Verification items for the finished model (mm, model axes). Face numbers are marked on the shaded views. A direction names the side the tool comes from. Coordinates: 2 decimals unless noted, no trailing zeros. Write each loop counter-clockwise with the first axis right and the second up, starting at its lowest first coordinate (ties: lowest second). Pieces come first, ordered by that corner, then holes. Notation, with made-up numbers: (85, 82.5) -> (126, 82.5) arc R21 cw to (126, 121.5) -> close; hole circle Ø5 at (79, 7). An arc over 180 degrees is marked (long way). Use CSV: the item, a comma, the result in double quotes.
```python
from build123d import *

# Parameters (mm, degrees)
SKETCH1_W                 = 200
SKETCH1_H                 = 177.5
BOSS_EXTRUDE1_DEPTH       = 2.5
BOSS_EXTRUDE2_DEPTH       = 40
SKETCH5_W                 = 86.25
SKETCH5_H                 = 95
BOSS_EXTRUDE3_DEPTH       = 2.5
CUT_EXTRUDE1_DEPTH        = 285.62694883
CUT_EXTRUDE1_DEPTH_BACK   = 285.62694883
BOSS_EXTRUDE4_START       = -177.5
BOSS_EXTRUDE4_DEPTH       = 177.5
SKETCH9_W                 = 167.5
SKETCH9_H                 = 15
CUT_EXTRUDE2_DEPTH        = 285.62694883
SKETCH15_R                = 2.65
CUT_EXTRUDE5_DEPTH        = 10
LPATTERN1_COUNT           = 4
LPATTERN1_PITCH           = 17.5
LPATTERN2_COUNT           = 3
LPATTERN2_PITCH           = 20
LPATTERN2_COPY_1_SKETCH_R = 2.65
LPATTERN2_COPY_1_DEPTH    = 10
LPATTERN2_COPY_2_SKETCH_R = 2.65
LPATTERN2_COPY_2_DEPTH    = 10
LPATTERN2_COPY_3_SKETCH_R = 2.65
LPATTERN2_COPY_3_DEPTH    = 10
LPATTERN2_COPY_4_SKETCH_R = 2.65
LPATTERN2_COPY_4_DEPTH    = 10
LPATTERN2_COPY_5_SKETCH_R = 2.65
LPATTERN2_COPY_5_DEPTH    = 10
LPATTERN2_COPY_6_SKETCH_R = 2.65
LPATTERN2_COPY_6_DEPTH    = 10
SKETCH16_W                = 90
SKETCH16_H                = 60
CUT_EXTRUDE6_DEPTH        = 10


# Read off the part's stored shape, not the designer's step: Boss-Extrude2
with BuildPart() as part:
    # Sketch1 → Boss-Extrude1 (new body)
    with BuildSketch(Plane(origin=(0, 0, 0), x_dir=(0, 1, 0), z_dir=(0, 0, 1))):
        with Locations((100, 88.75)):
            Rectangle(SKETCH1_W, SKETCH1_H)
    extrude(amount=BOSS_EXTRUDE1_DEPTH)

    # Boss-Extrude2 outline → Boss-Extrude2 (add)
    with BuildSketch(Plane.XY.offset(2.5)):
        Polygon((-177.5, 143.75), (-177.5, 0), (0, 0), (0, 143.75), (-2.5, 143.75), (-2.5, 2.5), (-175, 2.5), (-175, 143.75), align=None)
    extrude(amount=BOSS_EXTRUDE2_DEPTH)

    # Sketch5 → Boss-Extrude3 (add)
    with BuildSketch(Plane.YZ):
        with Locations((156.875, 50)):
            Rectangle(SKETCH5_W, SKETCH5_H)
    boss_extrude3 = extrude(amount=-BOSS_EXTRUDE3_DEPTH)

    # Mirror2: Boss-Extrude3 across plane
    add(boss_extrude3.mirror(Plane(origin=(-88.75, 0, 0), x_dir=(0, 0, 1), z_dir=(1, 0, 0))))

    # Sketch6 → Cut-Extrude1 (cut, two sides: drawn at the far end of the back side and taken through both)
    with BuildSketch(Plane.YZ.offset(-CUT_EXTRUDE1_DEPTH_BACK)):
        Polygon((113.75, 97.5), (113.75, 42.5), (180, 97.5), align=None)
    extrude(amount=CUT_EXTRUDE1_DEPTH + CUT_EXTRUDE1_DEPTH_BACK, mode=Mode.SUBTRACT)

    # Sketch7 → Boss-Extrude4 (add)
    with BuildSketch(Plane.YZ.offset(BOSS_EXTRUDE4_START)):
        Polygon((113.75, 47.5), (113.75, 42.5), (123.75, 42.5), (123.75, 47.5), (184.943404756, 93.683701702), (200, 93.683701702), (200, 97.5), (180, 97.5), align=None)
    extrude(amount=BOSS_EXTRUDE4_DEPTH)

    # Sketch9 → Cut-Extrude2 (cut, through all)
    with BuildSketch(Plane.XZ):
        with Locations((-88.75, 35)):
            Rectangle(SKETCH9_W, SKETCH9_H)
    extrude(amount=-CUT_EXTRUDE2_DEPTH, mode=Mode.SUBTRACT)

    # Sketch15 → Cut-Extrude5 (cut)
    with BuildSketch(Plane(origin=(0, 18.439555455, -24.432410978), x_dir=(1, 0, 0), z_dir=(0, -0.6024069059118725, 0.7981891503332306))):
        with Locations(Location((-157.5, 188.315762576, 0), (0, 0, 270))):
            Circle(SKETCH15_R)
    cut_extrude5 = extrude(amount=-CUT_EXTRUDE5_DEPTH, mode=Mode.SUBTRACT)

    # LPattern1: Cut-Extrude5 ×4
    with Locations(*[Vector(0, -0.7981891503332306, -0.6024069059118724) * (i * LPATTERN1_PITCH) for i in range(1, LPATTERN1_COUNT)]):
        add(cut_extrude5, mode=Mode.SUBTRACT)

    # LPattern2: Cut-Extrude5 ×3
    with Locations(*[(i * LPATTERN2_PITCH, 0, 0) for i in range(1, LPATTERN2_COUNT)]):
        add(cut_extrude5, mode=Mode.SUBTRACT)

    # LPattern2 copy 1 sketch → LPattern2 copy 1 (cut)
    with BuildSketch(Plane(origin=(20, 4.471245324, -34.974531831), x_dir=(1, 0, 0), z_dir=(0, -0.6024069059118725, 0.7981891503332306))):
        with Locations(Location((-157.5, 188.315762576, 0), (0, 0, 270))):
            Circle(LPATTERN2_COPY_1_SKETCH_R)
    extrude(amount=-LPATTERN2_COPY_1_DEPTH, mode=Mode.SUBTRACT)

    # LPattern2 copy 2 sketch → LPattern2 copy 2 (cut)
    with BuildSketch(Plane(origin=(40, 4.471245324, -34.974531831), x_dir=(1, 0, 0), z_dir=(0, -0.6024069059118725, 0.7981891503332306))):
        with Locations(Location((-157.5, 188.315762576, 0), (0, 0, 270))):
            Circle(LPATTERN2_COPY_2_SKETCH_R)
    extrude(amount=-LPATTERN2_COPY_2_DEPTH, mode=Mode.SUBTRACT)

    # LPattern2 copy 3 sketch → LPattern2 copy 3 (cut)
    with BuildSketch(Plane(origin=(20, -9.497064807, -45.516652684), x_dir=(1, 0, 0), z_dir=(0, -0.6024069059118725, 0.7981891503332306))):
        with Locations(Location((-157.5, 188.315762576, 0), (0, 0, 270))):
            Circle(LPATTERN2_COPY_3_SKETCH_R)
    extrude(amount=-LPATTERN2_COPY_3_DEPTH, mode=Mode.SUBTRACT)

    # LPattern2 copy 4 sketch → LPattern2 copy 4 (cut)
    with BuildSketch(Plane(origin=(40, -9.497064807, -45.516652684), x_dir=(1, 0, 0), z_dir=(0, -0.6024069059118725, 0.7981891503332306))):
        with Locations(Location((-157.5, 188.315762576, 0), (0, 0, 270))):
            Circle(LPATTERN2_COPY_4_SKETCH_R)
    extrude(amount=-LPATTERN2_COPY_4_DEPTH, mode=Mode.SUBTRACT)

    # LPattern2 copy 5 sketch → LPattern2 copy 5 (cut)
    with BuildSketch(Plane(origin=(20, -23.465374938, -56.058773538), x_dir=(1, 0, 0), z_dir=(0, -0.6024069059118725, 0.7981891503332306))):
        with Locations(Location((-157.5, 188.315762576, 0), (0, 0, 270))):
            Circle(LPATTERN2_COPY_5_SKETCH_R)
    extrude(amount=-LPATTERN2_COPY_5_DEPTH, mode=Mode.SUBTRACT)

    # LPattern2 copy 6 sketch → LPattern2 copy 6 (cut)
    with BuildSketch(Plane(origin=(40, -23.465374938, -56.058773538), x_dir=(1, 0, 0), z_dir=(0, -0.6024069059118725, 0.7981891503332306))):
        with Locations(Location((-157.5, 188.315762576, 0), (0, 0, 270))):
            Circle(LPATTERN2_COPY_6_SKETCH_R)
    extrude(amount=-LPATTERN2_COPY_6_DEPTH, mode=Mode.SUBTRACT)

    # Sketch16 → Cut-Extrude6 (cut)
    with BuildSketch(Plane(origin=(0, 18.439555455, -24.432410978), x_dir=(1, 0, 0), z_dir=(0, -0.6024069059118724, 0.7981891503332307))):
        with Locations((-55, 163.315762576)):
            Rectangle(SKETCH16_W, SKETCH16_H)
    extrude(amount=-CUT_EXTRUDE6_DEPTH, mode=Mode.SUBTRACT)


solid = part.part
```
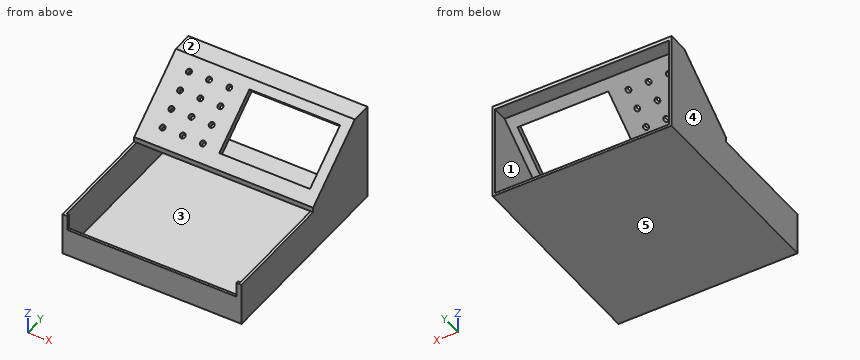
1) Cross-section at D-D (z = 21.5). Record the boundary of the cut face in (x, y), plus the area to 3 significant figures.
Return value:
outline,"(-177.5, 0) -> (0, 0) -> (0, 200) -> (-2.5, 200) -> (-2.5, 2.5) -> (-175, 2.5) -> (-175, 200) -> (-177.5, 200) -> close"
area,"1,430 mm2"
2) Cross-section at C-C (y = 90). Record the boundary of the cut face in (x, z), plus the area to 3 significant figures.
Return value:
outline,"(-177.5, 0) -> (0, 0) -> (0, 42.5) -> (-2.5, 42.5) -> (-2.5, 2.5) -> (-175, 2.5) -> (-175, 42.5) -> (-177.5, 42.5) -> close"
area,"644 mm2"
3) Mould release check, pull along Z, two halves, no side actions. Record for the marked faces 3, 4 and 5: released by +Z, released by -Z, zero draft, split by the parting line, or undercut.
Return value:
face 3,"undercut"
face 4,"zero draft"
face 5,"released by -Z"
4) Cross-section at B-B (x = -13). Record the boundary of the cut face in (y, z).
Return value:
outline,"(0, 0) -> (200, 0) -> (200, 2.5) -> (2.5, 2.5) -> (2.5, 27.5) -> (0, 27.5) -> close; (113.75, 42.5) -> (123.75, 42.5) -> (123.75, 47.5) -> (128.48, 51.07) -> (124.85, 55.88) -> (113.75, 47.5) -> close; (172.74, 92.02) -> (176.37, 87.21) -> (184.94, 93.68) -> (200, 93.68) -> (200, 97.5) -> (180, 97.5) -> close"
5) Cross-section at A-A (x = -104). Record the boundary of the cut face in (y, z), plus the area to 3 significant figures.
Return value:
outline,"(0, 0) -> (200, 0) -> (200, 2.5) -> (2.5, 2.5) -> (2.5, 27.5) -> (0, 27.5) -> close; (113.75, 42.5) -> (123.75, 42.5) -> (123.75, 47.5) -> (184.94, 93.68) -> (200, 93.68) -> (200, 97.5) -> (180, 97.5) -> (113.75, 47.5) -> close"
area,"1,160 mm2"
6) Scan lines: L1, parallel to X at y = 166.5, z = 34.5; L2, parallel to Z at x = -101, y = 52. Record each from-to range of solid material in increasing order.
Return value:
L1,"-177.5 to -175, -2.5 to 0"
L2,"0 to 2.5"
7) Set-up check for the marked faces 1 and 2: record each of +Z, -Z, +X, -X, +Y, -Y from which the full face is reachable in a straight line by a thin tool's end or side.
Return value:
face 1,"+Y"
face 2,"+Z, +X, -X, +Y, -Y"
8) Gauge pin test, flat ends, axial feed: pin 1 (5.5 mm diameter, centred on x = -128, z = 45.5, fed in from -Y); pin 2 (12 mm diameter, centred on x = -154.5, y = 124.5, fed in from +Z); pin 3 (4 mm diameter, centred on x = -58, z = 44.5, fed in from +Y). Record the tip position at first contact, or that the pin passes through.
Return value:
pin 1,"y = 113.75"
pin 2,"z = 60.14"
pin 3,"y = 123.75"
